Work out the finished part from the listing and answer in its coordinate system (mm). Give positions to 0.01 mm unless a question says otherwise; leave off trailing zeros. Order: outer loops, then holes, each group sorted by start corner. A loop starts at its lowest first (then second) coordinate and runs counter-clockwise, first axis right, second up. Notation, with made-up numbers: (-22, 61) - (32, 61) arc R31 ccw to (32, 98) - close; hole circle Ø10 at (31, -34.5). An arc over 180 degrees is marked (long way). Write each question's results on one line, items separated by ' | '.
from build123d import *

# Parameters (mm, degrees)
SKETCH1_R          = 11.1125
BASE_FLANGE1_DEPTH = 3.175
SKETCH2_R          = 3.175
TAB1_DEPTH         = 3.175
SKETCH3_R          = 3.175
CUT_EXTRUDE1_DEPTH = 209.903242457
FILLET1_R          = 1.5875


# Sheet-metal steps are written as plain solids
with BuildPart() as part:
    # Sketch1 → Base-Flange1 (new body)
    with BuildSketch(Plane(origin=(0, 0, 0), x_dir=(0, 0, -1), z_dir=(1, 0, 0))):
        with BuildLine():
            Line((0, 0), (0, 25.4))
            Line((0, 25.4), (-39.085182146, 66.301387632))
            ThreePointArc((-39.085182146, 66.301387632), (-41.252321544, 89.894394258), (-18.764209654, 97.351691251))
            Line((-18.764209654, 97.351691251), (177.8, 25.4))
            Line((177.8, 25.4), (177.8, 0))
            Line((177.8, 0), (0, 0))
        make_face()
        with Locations((-25.3124843, 79.462515777)):
            Circle(SKETCH1_R, mode=Mode.SUBTRACT)
    extrude(amount=-BASE_FLANGE1_DEPTH)

    # Sketch2 → Tab1 (add)
    with BuildSketch(Plane(origin=(0, 0, 0), x_dir=(0, 0, -1), z_dir=(1, 0, 0))):
        with BuildLine():
            Line((-46.659727461, 109.126939283), (-18.616317191, 97.313010257))
            ThreePointArc((-18.616317191, 97.313010257), (-18.335147008, 97.198498454), (-18.051319944, 97.090740286))
            Line((-18.051319944, 97.090740286), (-18.764209654, 97.351691251))
            ThreePointArc((-18.764209654, 97.351691251), (-39.101007237, 92.607063514), (-42.868254817, 72.06674526))
            Line((-42.868254817, 72.06674526), (-54.976907806, 100.809758938))
            ThreePointArc((-54.976907806, 100.809758938), (-53.615112361, 107.765143837), (-46.659727461, 109.126939283))
        make_face()
        with Locations((-49.1249843, 103.275015777)):
            Circle(SKETCH2_R, mode=Mode.SUBTRACT)
    extrude(amount=-TAB1_DEPTH)

    # Sketch3 → Cut-Extrude1 (cut, through all)
    with BuildSketch(Plane.ZY.offset(3.175)):
        with Locations((-95.25, 12.7)):
            Circle(SKETCH3_R)
        with Locations((-12.7, 12.7)):
            Circle(SKETCH3_R)
        with Locations((-44.45, 12.7)):
            Circle(SKETCH3_R)
        with BuildLine():
            Line((-107.95, 25.4), (-107.95, 0))
            Line((-107.95, 0), (-177.8, 0))
            Line((-177.8, 0), (-177.8, 25.4))
            Line((-177.8, 25.4), (-83.93965963, 59.757273091))
            ThreePointArc((-83.93965963, 59.757273091), (-101.35258254, 46.357806773), (-107.95, 25.4))
        make_face()
    extrude(amount=-CUT_EXTRUDE1_DEPTH, mode=Mode.SUBTRACT)

    # Fillet1
    fillet1_edges = [part.edges().sort_by_distance(p)[0] for p in [
        (-1.5875, 25.4, 0),
    ]]
    fillet(fillet1_edges, radius=FILLET1_R)


solid = part.part
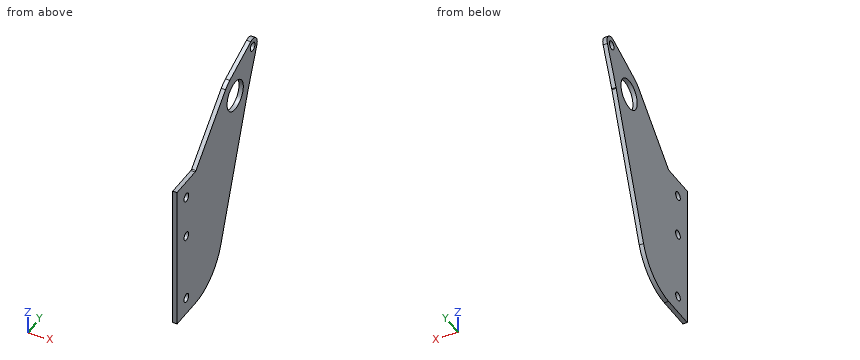
1. A cutting plane is placed at A-A, the plane z = 29.5. Write down the section's boundary in (x, y) (3 decimals), then the cut area to 3 significant figures.
Answer list:
outline: (-3.175, 56.271) - (0, 56.271) - (0, 69.169) - (-3.175, 69.169) - close; (-3.175, 89.756) - (0, 89.756) - (0, 101.898) - (-3.175, 101.898) - close | area: 79.5 mm^2
2. A cutting plane is placed at D-D, the plane y = 39. Write down the section's boundary in (x, z) (3 decimals), then the cut area to 3 significant figures.
Answer list:
outline: (-3.175, -105.328) - (0, -105.328) - (0, 12.996) - (-3.175, 12.996) - close | area: 376 mm^2
3. Given P1, Ø1.5, axis at x = -0.5, z = -64, coming from the -Y side; P2, Ø1.6, axis at x = -1, y = 16.5, coming from the +Z side, each flat-ended and moving along its own axis, determine where each tip first touches the part or whether it passes through.
Answer list:
P1: y = 0 | P2: z = 0
4. A cutting plane is placed at C-C, the plane x = -2.45. State how many separate pieces and enclosed holes the cut face has, then the cut area to 3 significant figures.
Answer list:
separate pieces: 1 | enclosed holes: 5 | area: 9,450 mm^2
5. Straight lines are drawn through the part: line 1 (Z direction, x = -2.7, y = 19.5); line 2 (Y direction, x = -1.2, z = -45); line 3 (Y direction, x = -1.45, z = -94). For each, find the intervals that lie inside material, in ascending order. Write a range as [from, to].
Answer list:
line 1: [-107.95, 0] | line 2: [0, 9.57], [15.83, 74.01] | line 3: [0, 9.78], [15.62, 54.14]
6. A cutting plane is placed at B-B, the plane y = 75.5. Write down the section's boundary in (x, z) (1 decimal).
Answer list:
outline: (-3.2, -40.9) - (0, -40.9) - (0, 14.9) - (-3.2, 14.9) - close; (-3.2, 35.7) - (0, 35.7) - (0, 44.3) - (-3.2, 44.3) - close
